The listing builds one solid part. Answer for the finished solid, in the listing's coordinates (mm). Give positions to 0.01 mm unless a question says otherwise; leave off trailing zeros. Loops run counter-clockwise (first coordinate to the right, second up) from the corner with the lowest first, then second, coordinate; pieces in that order, holes last. Notation, with made-up numbers: (87, 34) -> (144, 34) arc R21 cw to (144, 55) -> close; hole circle Ø7 at (34.5, -9). An arc over 180 degrees is marked (long way). One line per question, with ' | ' between items. Start each with the question number.
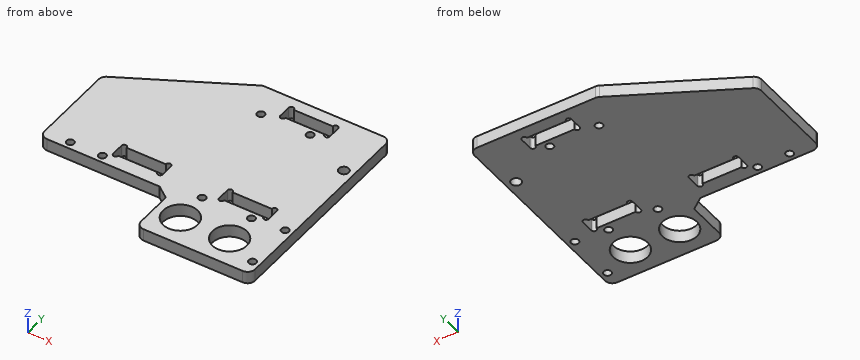
from build123d import *

# Parameters (mm, degrees)
EXTRUDE_1_DEPTH           = 5
SKETCH_4_W                = 20.1
SKETCH_4_H                = 5.1
CUT_EXTRUDE_3_DEPTH       = 1
CUT_EXTRUDE_3_DEPTH_BACK  = 6
CUT_EXTRUDE_4_DEPTH       = 6
SKETCH_6_R                = 1.525
CUT_EXTRUDE_5_DEPTH       = 1
CUT_EXTRUDE_5_DEPTH_BACK  = 6
CUT_EXTRUDE_6_DEPTH       = 1
CUT_EXTRUDE_6_DEPTH_BACK  = 6
SKETCH_8_W                = 53.737387097
SKETCH_8_H                = 38.025
EXTRUDE_2_DEPTH           = 5
SKETCH_11_R               = 1.525
CUT_EXTRUDE_9_DEPTH       = 1
CUT_EXTRUDE_9_DEPTH_BACK  = 6
SKETCH_14_R               = 2.025
CUT_EXTRUDE_10_DEPTH      = 10
SKETCH_15_W               = 2.1
SKETCH_15_H               = 5.1
SKETCH_15_W_2             = 15.9
CUT_EXTRUDE_11_DEPTH      = 6
SKETCH_16_R               = 1.525
CUT_EXTRUDE_12_DEPTH      = 1
CUT_EXTRUDE_12_DEPTH_BACK = 6
CUT_EXTRUDE_13_DEPTH      = 10
EXTRUDE_3_DEPTH           = 5
EXTRUDE_4_DEPTH           = 5
FILLET_1_R                = 3
SKETCH_20_R               = 7
CUT_EXTRUDE_14_DEPTH      = 5
SKETCH_21_R               = 1.525
CUT_EXTRUDE_15_DEPTH      = 8
CUT_EXTRUDE_17_DEPTH      = 6


with BuildPart() as part:
    # 草图1 → 凸台-拉伸1 (new body)
    with BuildSketch(Plane.XY):
        Polygon((0, 0), (-46.262612903, 16.838214056), (-46.262612903, 27.95), (-86.262612903, 27.95), (-100, 32.95), (-100, 87), (0, 87), align=None)
    extrude(amount=EXTRUDE_1_DEPTH)

    # 草图4 → 切除-拉伸3 (cut, two sides)
    with BuildSketch(Plane(origin=(0, 0, 0), x_dir=(-1, 0, 0), z_dir=(0, 0, -1))) as cut_extrude_3_sk:
        with Locations((28, 78.5)):
            Rectangle(SKETCH_4_W, SKETCH_4_H)
    extrude(amount=CUT_EXTRUDE_3_DEPTH, mode=Mode.SUBTRACT)
    extrude(cut_extrude_3_sk.sketch, amount=-CUT_EXTRUDE_3_DEPTH_BACK, mode=Mode.SUBTRACT)

    # 草图5 → 切除-拉伸4 (cut, through all)
    with BuildSketch(Plane(origin=(0, 0, 0), x_dir=(-1, 0, 0), z_dir=(0, 0, -1))):
        with BuildLine():
            Line((38.05, 81.05), (38.05, 75.95))
            ThreePointArc((38.05, 75.95), (37, 74.9), (35.95, 75.95))
            Line((35.95, 75.95), (35.95, 81.05))
            ThreePointArc((35.95, 81.05), (37, 82.1), (38.05, 81.05))
        make_face()
        with BuildLine():
            Line((17.95, 81.05), (17.95, 75.95))
            ThreePointArc((17.95, 75.95), (19, 74.9), (20.05, 75.95))
            Line((20.05, 75.95), (20.05, 81.05))
            ThreePointArc((20.05, 81.05), (19, 82.1), (17.95, 81.05))
        make_face()
    extrude(amount=-CUT_EXTRUDE_4_DEPTH, mode=Mode.SUBTRACT)

    # 草图6 → 切除-拉伸5 (cut, two sides)
    with BuildSketch(Plane(origin=(0, 0, 0), x_dir=(-1, 0, 0), z_dir=(0, 0, -1))) as cut_extrude_5_sk:
        with Locations((23.96256416, 73)):
            Circle(SKETCH_6_R)
        with Locations((43.96256416, 73)):
            Circle(SKETCH_6_R)
    extrude(amount=CUT_EXTRUDE_5_DEPTH, mode=Mode.SUBTRACT)
    extrude(cut_extrude_5_sk.sketch, amount=-CUT_EXTRUDE_5_DEPTH_BACK, mode=Mode.SUBTRACT)

    # 草图7 → 切除-拉伸6 (cut, two sides)
    with BuildSketch(Plane(origin=(0, 0, 0), x_dir=(-1, 0, 0), z_dir=(0, 0, -1))) as cut_extrude_6_sk:
        Polygon((50, 87), (100, 59.975), (100, 87), align=None)
    extrude(amount=CUT_EXTRUDE_6_DEPTH, mode=Mode.SUBTRACT)
    extrude(cut_extrude_6_sk.sketch, amount=-CUT_EXTRUDE_6_DEPTH_BACK, mode=Mode.SUBTRACT)

    # 草图8 → 凸台-拉伸2 (add)
    with BuildSketch(Plane(origin=(0, 0, 0), x_dir=(-1, 0, 0), z_dir=(0, 0, -1))):
        with Locations((73.131306451, 40.9625)):
            Rectangle(SKETCH_8_W, SKETCH_8_H)
    extrude(amount=-EXTRUDE_2_DEPTH)

    # 草图11 → 切除-拉伸9 (cut, two sides)
    with BuildSketch(Plane.XY.offset(5)) as cut_extrude_9_sk:
        with Locations((-3, 6)):
            Circle(SKETCH_11_R)
        with Locations((-3, 26)):
            Circle(SKETCH_11_R)
    extrude(amount=CUT_EXTRUDE_9_DEPTH, mode=Mode.SUBTRACT)
    extrude(cut_extrude_9_sk.sketch, amount=-CUT_EXTRUDE_9_DEPTH_BACK, mode=Mode.SUBTRACT)

    # 草图14 → 切除-拉伸10 (cut)
    with BuildSketch(Plane(origin=(0, 0, 0), x_dir=(-1, 0, 0), z_dir=(0, 0, -1))):
        with Locations((4, 63.499999999)):
            Circle(SKETCH_14_R)
    extrude(amount=-CUT_EXTRUDE_10_DEPTH, mode=Mode.SUBTRACT)

    # 草图15 → 切除-拉伸11 (cut, through all)
    with BuildSketch(Plane(origin=(0, 0, 0), x_dir=(-1, 0, 0), z_dir=(0, 0, -1))):
        with BuildLine():
            ThreePointArc((56.05, 33), (55, 34.05), (53.95, 33))
            Line((53.95, 33), (56.05, 33))
        make_face()
        with Locations((55, 30.45)):
            Rectangle(SKETCH_15_W, SKETCH_15_H)
        with Locations((64, 30.45)):
            Rectangle(SKETCH_15_W_2, SKETCH_15_H)
        with BuildLine():
            Line((56.05, 27.9), (53.95, 27.9))
            ThreePointArc((53.95, 27.9), (55, 26.85), (56.05, 27.9))
        make_face()
        with BuildLine():
            ThreePointArc((74.05, 33), (73, 34.05), (71.95, 33))
            Line((71.95, 33), (74.05, 33))
        make_face()
        with Locations((73, 30.45)):
            Rectangle(SKETCH_15_W, SKETCH_15_H)
        with BuildLine():
            Line((74.05, 27.9), (71.95, 27.9))
            ThreePointArc((71.95, 27.9), (73, 26.85), (74.05, 27.9))
        make_face()
        with Locations((12, 30.45)):
            Rectangle(SKETCH_15_W, SKETCH_15_H)
        with BuildLine():
            Line((13.05, 27.9), (10.95, 27.9))
            ThreePointArc((10.95, 27.9), (12, 26.85), (13.05, 27.9))
        make_face()
        with Locations((21, 30.45)):
            Rectangle(SKETCH_15_W_2, SKETCH_15_H)
        with BuildLine():
            ThreePointArc((13.05, 33), (12, 34.05), (10.95, 33))
            Line((10.95, 33), (13.05, 33))
        make_face()
        with Locations((30, 30.45)):
            Rectangle(SKETCH_15_W, SKETCH_15_H)
        with BuildLine():
            Line((31.05, 27.9), (28.95, 27.9))
            ThreePointArc((28.95, 27.9), (30, 26.85), (31.05, 27.9))
        make_face()
        with BuildLine():
            ThreePointArc((31.05, 33), (30, 34.05), (28.95, 33))
            Line((28.95, 33), (31.05, 33))
        make_face()
    extrude(amount=-CUT_EXTRUDE_11_DEPTH, mode=Mode.SUBTRACT)

    # 草图16 → 切除-拉伸12 (cut, two sides)
    with BuildSketch(Plane(origin=(0, 0, 0), x_dir=(-1, 0, 0), z_dir=(0, 0, -1))) as cut_extrude_12_sk:
        with Locations((16, 24.95)):
            Circle(SKETCH_16_R)
        with Locations((36, 24.95)):
            Circle(SKETCH_16_R)
    extrude(amount=CUT_EXTRUDE_12_DEPTH, mode=Mode.SUBTRACT)
    extrude(cut_extrude_12_sk.sketch, amount=-CUT_EXTRUDE_12_DEPTH_BACK, mode=Mode.SUBTRACT)

    # 草图17 → 切除-拉伸13 (cut)
    with BuildSketch(Plane(origin=(0, 0, 0), x_dir=(-1, 0, 0), z_dir=(0, 0, -1))):
        Polygon((0, 86), (51.85013876, 86), (50, 87), (0, 87), align=None)
    extrude(amount=-CUT_EXTRUDE_13_DEPTH, mode=Mode.SUBTRACT)

    # 草图18 → 凸台-拉伸3 (add)
    with BuildSketch(Plane.XY.offset(5)):
        Polygon((-46.262612903, 16.838214056), (-46.262612903, 0), (0, 0), align=None)
    extrude(amount=-EXTRUDE_3_DEPTH)

    # 草图19 → 凸台-拉伸4 (add)
    with BuildSketch(Plane.XY.offset(5)):
        Polygon((-46.262612903, 6.95), (-66.262612903, 21.95), (-46.262612903, 21.95), align=None)
    extrude(amount=-EXTRUDE_4_DEPTH)

    # 圆角1
    fillet_1_edges = [part.edges().sort_by_distance(p)[0] for p in [
        (-100, 21.95, 2.5),
        (0, 0, 2.5),
        (-51.85013876, 86, 2.5),
        (0, 86, 2.5),
        (-46.262612903, 0, 2.5),
        (-100, 59.975, 2.5),
    ]]
    fillet(fillet_1_edges, radius=FILLET_1_R)

    # 草图20 → 切除-拉伸14 (cut)
    with BuildSketch(Plane.XY.offset(5)):
        with Locations((-36.262612903, 12)):
            Circle(SKETCH_20_R)
        with Locations((-16.262612903, 12)):
            Circle(SKETCH_20_R)
    extrude(amount=-CUT_EXTRUDE_14_DEPTH, mode=Mode.SUBTRACT)

    # 草图21 → 切除-拉伸15 (cut)
    with BuildSketch(Plane.XY.offset(5)):
        with Locations((-89.5, 24.95)):
            Circle(SKETCH_21_R)
        with Locations((-76.5, 24.95)):
            Circle(SKETCH_21_R)
    extrude(amount=-CUT_EXTRUDE_15_DEPTH, mode=Mode.SUBTRACT)

    # 草图23 → 切除-拉伸17 (cut, through all)
    with BuildSketch(Plane(origin=(0, 0, 0), x_dir=(-1, 0, 0), z_dir=(0, 0, -1))):
        Polygon((46.262612903, 18.2), (46.262612903, 6.95), (66.262612903, 21.95), (51.262612903, 21.95), align=None)
    extrude(amount=-CUT_EXTRUDE_17_DEPTH, mode=Mode.SUBTRACT)


solid = part.part
1. Each of these flat-tipped pins is pushed along its axis until it touches: pin 1 Ø1.5 at (y, z) = (10, 3.5) entering from -X; pin 2 Ø1.5 at (x, y) = (-56.5, 31) entering from +Z. Where does it stop, or does it pass through?
2. The part is cut by section C-C (y = 30). Write down the section's boundary in (x, z), plus the area to 3 significant figures.
3. The part is cut by section A-A (y = 12). Write down the section's boundary in (x, z), plus the area to 3 significant figures.
4. The part is cut by section B-B (x = -76.5). Write down the section's boundary in (y, z) (3 decimals), plus the area to 3 significant figures.
5. The part is cut by section D-D (z = 3.1). Count the separate pieces of the cut face and the enclosed holes in it, plus the area to 3 significant figures.
6. Straight lines are drawn through the part: L1, parallel to X at y = 28, z = 3.5; L2, parallel to X at y = 11.5, z = 0.85; L3, parallel to Y at x = -15, z = 4. For each, find the intervals that lie inside material, in ascending order.
Check sheet entries:
1) pin 1: stops at x = -46.26 | pin 2: passes through
2) outline: (-100, 0) -> (-74.05, 0) -> (-74.05, 5) -> (-100, 5) -> close; (-53.95, 0) -> (-31.05, 0) -> (-31.05, 5) -> (-53.95, 5) -> close; (-10.95, 0) -> (0, 0) -> (0, 5) -> (-10.95, 5) -> close | area: 299 mm^2
3) outline: (-46.26, 0) -> (-43.26, 0) -> (-43.26, 5) -> (-46.26, 5) -> close; (-29.26, 0) -> (-23.26, 0) -> (-23.26, 5) -> (-29.26, 5) -> close; (-9.26, 0) -> (0, 0) -> (0, 5) -> (-9.26, 5) -> close | area: 91.3 mm^2
4) outline: (21.95, 0) -> (23.425, 0) -> (23.425, 5) -> (21.95, 5) -> close; (26.475, 0) -> (72.677, 0) -> (72.677, 5) -> (26.475, 5) -> close | area: 238 mm^2
5) separate pieces: 1 | enclosed holes: 14 | area: 6,090 mm^2
6) L1: x = -100 to -74.05, -53.95 to -31.05, -10.95 to 0 | L2: x = -46.26 to -43.24, -29.28 to -23.24, -9.28 to 0 | L3: y = 0 to 5.11, 18.89 to 23.8, 26.1 to 27.9, 33 to 86
